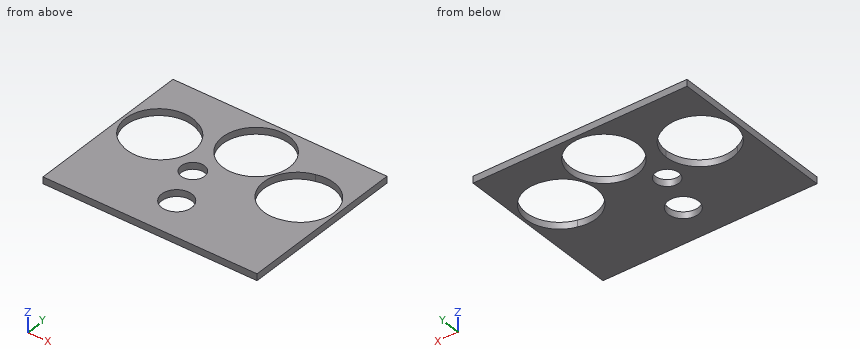
Autodesk Inventor part; units mm, degrees
ref_plane "YZ Plane" through (0, 0, 0) normal (1, 0, 0) x (0, 1, 0)
ref_plane "XZ Plane" through (0, 0, 0) normal (0, 1, 0) x (-1, 0, 0)
ref_plane "XY Plane" through (0, 0, 0) normal (0, 0, 1) x (1, 0, 0)
sketch "Sketch1" plane through (0, 0, 0) normal (0, 0, 1) x (1, 0, 0)
  line L0 (0, 0) -> (304.8, 0) construction
  line L1 (304.8, 0) -> (304.8, 50.8) construction
  line L2 (304.8, 50.8) -> (0, 50.8) construction
  line L3 (0, 50.8) -> (0, 0) construction
  circle A0 centre (152.4, 25.4) radius 14.2875
  circle A1 centre (152.4, 25.4) radius 30.48 construction
  circle A2 centre (152.4, 25.4) radius 22.225 construction
  line L4 (152.4, 25.4) -> (138.508178, 62.969727) construction
  circle A3 centre (138.508178, 62.969727) radius 9.525 construction
  circle A4 centre (138.508178, 62.969727) radius 17.78 construction
  circle A5 centre (89.971088, 85.09) radius 31.75 construction
  circle A6 centre (160.978478, 111.345767) radius 31.75
  circle A7 centre (221.970096, 85.09) radius 31.75 construction
  line L5 (0, 50.8) -> (0, 53.34) construction
  line L6 (0, 53.34) -> (304.8, 53.34) construction
  line L7 (304.8, 53.34) -> (304.8, 50.8) construction
  circle A8 centre (138.508178, 62.969727) radius 21.59 construction
  circle A9 centre (152.4, 25.4) radius 46.99 construction
  circle A10 centre (152.4, 25.4) radius 50.8 construction
  arc A11 (84.94082, 79.326416) -> (90.918413, 92.681118) centre (89.971088, 85.09) ccw construction
  circle A12 centre (160.978478, 111.345767) radius 7.65 construction
  arc A13 (221.694578, 92.735037) -> (225.517168, 78.312037) centre (221.970096, 85.09) ccw construction
  circle A14 centre (160.978478, 111.345767) radius 9.1 construction
  circle A15 centre (138.508178, 62.969727) radius 22.9 construction
  line L8 (84.94082, 79.326416) -> (123.450252, 45.716644) construction
  line L9 (168.548316, 110.241211) -> (161.168218, 59.663279) construction
  line L10 (90.918413, 92.681118) -> (89.971088, 85.09) construction
  line L11 (89.971088, 85.09) -> (84.94082, 79.326416) construction
  circle A16 centre (126.19198, 96.27826) radius 3.175 construction
  circle A17 centre (126.19198, 96.27826) radius 7.9375 construction
  line L12 (90.918413, 92.681118) -> (125.209053, 88.401855) construction
  line L13 (132.062639, 90.936044) -> (155.320457, 116.494485) construction
  line L14 (155.320457, 116.494485) -> (160.978478, 111.345767) construction
  line L15 (168.548316, 110.241211) -> (160.978478, 111.345767) construction
  line L16 (138.508178, 62.969727) -> (126.19198, 96.27826) construction
  line L17 (89.971088, 85.09) -> (160.978478, 111.345767) construction
  line L18 (152.4, 25.4) -> (89.971088, 85.09) construction
  line L19 (152.4, 25.4) -> (160.978478, 111.345767) construction
  circle A18 centre (126.19198, 96.27826) radius 9.2075 construction
  circle A19 centre (126.19198, 96.27826) radius 6.1595 construction
  arc A20 (90.918413, 92.681118) -> (84.94082, 79.326416) centre (89.971088, 85.09) ccw construction
  circle A21 centre (160.978478, 111.345767) radius 25.4 construction
  circle A22 centre (221.970096, 85.09) radius 25.4 construction
  line L20 (102.942353, 114.069454) -> (76.999823, 56.110546) construction
  circle A23 centre (89.971088, 85.09) radius 25.4 construction
  line L21 (213.836088, 115.780396) -> (230.104105, 54.399604) construction
  line L22 (54.411088, 146.905767) -> (257.611088, 146.905767)
  line L23 (257.611088, 146.905767) -> (257.611088, -11.844233)
  line L24 (257.611088, -11.844233) -> (54.411088, -11.844233)
  line L25 (54.411088, -11.844233) -> (54.411088, 146.905767)
  circle A24 centre (138.508178, 62.969727) radius 11.1125
  arc A25 (225.312875, 75.445533) -> (221.093638, 95.322667) centre (223.203256, 85.3841) ccw construction
  line L26 (220.753147, 84.734737) -> (228.477303, 60.537683) construction
  line L27 (223.203256, 85.3841) -> (228.477303, 60.537683) construction
  line L28 (220.753147, 84.734737) -> (213.028991, 108.931791) construction
  line L29 (223.203256, 85.3841) -> (217.92921, 110.230517) construction
  arc A26 (212.304851, 111.200264) -> (213.75313, 106.663317) centre (213.028991, 108.931791) ccw construction
  arc A27 (218.423652, 107.901165) -> (217.434768, 112.559869) centre (217.92921, 110.230517) ccw construction
  arc A28 (218.423652, 107.901165) -> (213.75313, 106.663317) centre (228.477303, 60.537683) ccw construction
  arc A29 (217.434768, 112.559869) -> (212.304851, 111.200264) centre (228.477303, 60.537683) ccw construction
  line L30 (213.028991, 108.931791) -> (212.304851, 111.200264) construction
  line L31 (217.92921, 110.230517) -> (217.434768, 112.559869) construction
  arc A30 (221.093638, 95.322667) -> (217.663484, 94.413558) centre (228.477303, 60.537683) ccw construction
  arc A31 (225.312875, 75.445533) -> (223.842809, 75.055915) centre (228.477303, 60.537683) ccw construction
  line L32 (102.635769, 107.180274) -> (91.114923, 84.543355) construction
  line L33 (79.594076, 61.906436) -> (88.801403, 85.578892) construction
  arc A32 (98.871917, 111.470639) -> (97.145543, 107.032054) centre (98.00873, 109.251347) ccw construction
  arc A33 (101.55569, 105.058063) -> (103.715849, 109.302485) centre (102.635769, 107.180274) ccw construction
  arc A34 (101.55569, 105.058063) -> (97.145543, 107.032054) centre (79.594076, 61.906436) ccw construction
  line L34 (98.00873, 109.251347) -> (98.871917, 111.470639) construction
  line L35 (102.635769, 107.180274) -> (103.715849, 109.302485) construction
  arc A35 (103.715849, 109.302485) -> (98.871917, 111.470639) centre (79.594076, 61.906436) ccw construction
  arc A36 (217.663484, 94.413558) -> (223.842809, 75.055915) centre (220.753147, 84.734737) ccw construction
  arc A37 (86.506584, 75.488588) -> (95.723261, 93.598123) centre (91.114923, 84.543355) ccw construction
  line L36 (88.801403, 85.578892) -> (98.00873, 109.251347) construction
  line L37 (91.114923, 84.543355) -> (79.594076, 61.906436) construction
  arc A38 (86.506584, 75.488588) -> (85.118472, 76.10991) centre (79.594076, 61.906436) ccw construction
  arc A39 (95.723261, 93.598123) -> (92.484334, 95.047874) centre (79.594076, 61.906436) ccw construction
  arc A40 (92.484334, 95.047874) -> (85.118472, 76.10991) centre (88.801403, 85.578892) ccw construction
  line L38 (160.978478, 111.345767) -> (138.015112, 122.201357) construction
  line L39 (160.978478, 111.345767) -> (183.941843, 100.490177) construction
  circle A41 centre (138.508178, 62.969727) radius 26.75 construction
  line L40 (221.694578, 92.735037) -> (137.544764, 89.702373) construction
  line L41 (225.517168, 78.312037) -> (150.911337, 39.269007) construction
  line L42 (221.970096, 85.09) -> (221.694578, 92.735037) construction
  line L43 (221.970096, 85.09) -> (225.517168, 78.312037) construction
  line L44 (138.508178, 62.969727) -> (137.544764, 89.702373) construction
  line L45 (138.508178, 62.969727) -> (150.911337, 39.269007) construction
  arc A42 (225.517168, 78.312037) -> (221.694578, 92.735037) centre (221.970096, 85.09) ccw construction
  arc A43 (225.517168, 78.312037) -> (224.776319, 77.973286) centre (221.970096, 85.09) ccw construction
  line L46 (138.508178, 62.969727) -> (221.970096, 85.09) construction
  circle A44 centre (88.801403, 85.578892) radius 31.75
  circle A45 centre (91.114923, 84.543355) radius 31.75
  line L47 (98.871917, 111.470639) -> (100.310562, 115.16946) construction
  line L48 (103.715849, 109.302485) -> (105.515981, 112.839504) construction
  arc A46 (105.515981, 112.839504) -> (100.310562, 115.16946) centre (79.594076, 61.906436) ccw
  circle A47 centre (220.753147, 84.734737) radius 31.75
  circle A48 centre (223.203256, 85.3841) radius 31.75
  line L49 (212.304851, 111.200264) -> (211.097951, 114.981054) construction
  line L50 (217.434768, 112.559869) -> (216.610698, 116.442121) construction
  arc A49 (216.610698, 116.442121) -> (211.097951, 114.981054) centre (228.477303, 60.537683) ccw
  point P0 (215.46289, 109.642317)
  point P1 (100.3481, 108.273564)
  dimension "d114" = 63.5
  dimension "d115" = 63.5
  dimension "d122" = 63.5
  dimension "d123" = 63.5
  dimension "d1" = 50.8
  dimension "d2" = 28.575
  dimension "d3" = 25.4
  dimension "d4" = 152.4
  dimension "d7" = 60.96
  dimension "d8" = 44.45
  dimension "d9" = 19.05
  dimension "d10" = 35.56
  dimension "d11" = 40.0558
  dimension "d12" = 63.5
  dimension "d13" = 63.5
  dimension "d14" = 63.5
  dimension "d15" = 2.54
  dimension "d16" = 304.8
  dimension "d17" = 43.18
  dimension "d18" = 93.98
  dimension "d19" = 101.6
  dimension "d21" = 15.3
  dimension "d22" = 15.3
  dimension "d24" = 18.2
  dimension "d29" = 45.8
  dimension "d30" = 146
  dimension "d31" = 6.35
  dimension "d32" = 15.875
  dimension "d33" = 146
  dimension "d35" = 18.415
  dimension "d37" = 12.319
  dimension "d40" = 50.8
  dimension "d41" = 50.8
  dimension "d42" = 17
  dimension "d43" = 17
  dimension "d44" = 50.8
  dimension "d53" = 203.2
  dimension "d54" = 158.75
  dimension "d55" = 35.56
  dimension "d56" = 35.56
  dimension "d57" = 22.225
  dimension "d67" = 25.4
  dimension "d68" = 25.4
  dimension "d69" = 2.86
  dimension "d70" = 25.4
  dimension "d71" = 25.4
  dimension "d72" = 4.7625
  dimension "d75" = 2.86
  dimension "d80" = 4.7625
  dimension "d82" = 4.7625
  dimension "d83" = 50.8
  dimension "d84" = 50.8
  dimension "d85" = 10.16
  dimension "d97" = 48.41875
  dimension "d99" = 20.32
  dimension "d101" = 25.4
  dimension "d102" = 25.4
  dimension "d103" = 10.16
  dimension "d105" = 17
  dimension "d106" = 17
  dimension "d107" = 53.5
  dimension "d108" = 154.44
  dimension "d109" = 7.65
  dimension "d111" = 86.34349
  dimension "d112" = 12.7801
  dimension "d113" = 12.7801
  dimension "d116" = 57.15
sketch "Sketch1 outline for Extrusion3" plane through (0, 0, 0) normal (0, 0, 1) x (1, 0, 0)
  line L0 (54.411088, 146.905767) -> (257.611088, 146.905767)
  line L1 (54.411088, -11.844233) -> (54.411088, 146.905767)
  line L2 (257.611088, 146.905767) -> (257.611088, -11.844233)
  line L3 (257.611088, -11.844233) -> (54.411088, -11.844233)
  circle A0 centre (152.4, 25.4) radius 14.2875
  circle A1 centre (138.508178, 62.969727) radius 11.1125
  arc A2 (122.864923, 84.543355) -> (102.91909, 114.017482) centre (91.114923, 84.543355) ccw
  arc A3 (102.91909, 114.017482) -> (76.997235, 56.104765) centre (88.801403, 85.578892) ccw
  arc A4 (76.997235, 56.104765) -> (122.864923, 84.543355) centre (91.114923, 84.543355) ccw
  arc A5 (254.953256, 85.3841) -> (213.850676, 115.725355) centre (223.203256, 85.3841) ccw
  arc A6 (213.850676, 115.725355) -> (230.105727, 54.393482) centre (220.753147, 84.734737) ccw
  arc A7 (230.105727, 54.393482) -> (254.953256, 85.3841) centre (223.203256, 85.3841) ccw
  circle A8 centre (160.978478, 111.345767) radius 31.75
extrude "Extrusion3" add sketch "Sketch1 outline for Extrusion3" along normal blind 6.35
equation "\"d2\" = BearingLargeOD"
equation "\"d7\" = Gear48tPD"
equation "\"d8\" = Gear35tPD"
equation "\"d9\" = Gear15tPD"
equation "\"d10\" = Gear28tPD"
equation "\"d11\" = 0.5 * Gear48tPD + 0.5 * Gear15tPD + MeshingClearance"
equation "\"d12\" = CimOD"
equation "\"d13\" = CimOD"
equation "\"d14\" = CimOD"
equation "\"d17\" = Gear28tPD + ClearanceDiameter"
equation "\"d18\" = WheelOD"
equation "\"d19\" = WheelClearance"
equation "\"Pulley48tPD\" = 45.8"
equation "\"Pulley19tPD\" = 18.2"
equation "\"Pulley16tPD\" = 15.3"
equation "\"Gear15tPD\" = 19.05"
equation "\"Gear35tPD\" = 44.45"
equation "\"Gear48tPD\" = 60.96"
equation "\"Gear28tPD\" = 35.56"
equation "\"BearingLargeOD\" = 28.575"
equation "\"BearingSmallOD\" = 22.225"
equation "\"MeshingClearance\" = 0.0508"
equation "\"CimOD\" = 63.5"
equation "\"WheelOD\" = 93.98"
equation "\"ClearanceDiameter\" = 7.62"
equation "\"WheelClearance\" = 101.6"
equation "\"TensioningBearingID\" = 6.35"
equation "\"TensioningBearingOD\" = 15.875"
equation "\"SpingClipClearance\" = 8.89"
equation "\"Pi\" = 79.79645"
equation "\"Pulley56tPD\" = 53.5"
equation "\"BearingXLargeOD\" = 34.925"
properties part number "OutlineSketch1"
Verification items for the finished model (mm, model axes). Round coordinates to 2 decimals unless told otherwise and drop trailing zeros. Loops run counter-clockwise (first coordinate to the right, second up) from the corner with the lowest first, then second, coordinate; pieces in that order, holes last. Notation, with made-up numbers: (52, -6) - (79, -6) arc R11 cw to (79, -1) - close; hole circle Ø3 at (72.25, -9). An arc over 180 degrees is marked (long way). Use a Markdown table: item, result. Add a question column.
1. Section check C-C, the plane z = 3.75. Give the number of separate pieces and of enclosed holes in the cut face, plus the area to 3 significant figures.
2. Section check B-B, the plane x = 162. Record the boundary of the cut face in (y, z), plus the area to 3 significant figures.
3. Thickness scan on probe 1 along Y at (x, z) = (153, 3); probe 2 along X at (y, z) = (84, 5.75); probe 3 along Y at (x, z) = (152.4, 2). Record the ranges inside material, lowest first. Write a range as [from, to].
4. Section check D-D, the plane y = 76.5. Record the boundary of the cut face in (x, z), plus the area to 3 significant figures.
5. Section check A-A, the plane y = 25.4. Record the boundary of the cut face in (x, z).
Checks:
| question | item | result |
|---|---|---|
| 1 | separate pieces | 1 |
| 1 | enclosed holes | 5 |
| 1 | area | 21,400 mm^2 |
| 2 | outline | (-11.84, 0) - (14.82, 0) - (14.82, 6.35) - (-11.84, 6.35) - close; (35.98, 0) - (79.61, 0) - (79.61, 6.35) - (35.98, 6.35) - close; (143.08, 0) - (146.91, 0) - (146.91, 6.35) - (143.08, 6.35) - close |
| 2 | area | 471 mm^2 |
| 3 | probe 1 | y = [-11.84, 11.13], [39.67, 80.61], [142.08, 146.91] |
| 3 | probe 2 | x = [54.41, 57.09], [122.86, 144.85], [177.11, 189.01], [254.92, 257.61] |
| 3 | probe 3 | y = [-11.84, 11.11], [39.69, 80.78], [141.91, 146.91] |
| 4 | outline | (54.41, 0) - (58.38, 0) - (58.38, 6.35) - (54.41, 6.35) - close; (121.83, 0) - (190.09, 0) - (190.09, 6.35) - (121.83, 6.35) - close; (253.68, 0) - (257.61, 0) - (257.61, 6.35) - (253.68, 6.35) - close |
| 4 | area | 484 mm^2 |
| 5 | outline | (54.41, 0) - (138.11, 0) - (138.11, 6.35) - (54.41, 6.35) - close; (166.69, 0) - (257.61, 0) - (257.61, 6.35) - (166.69, 6.35) - close |
